Read the model definition and answer for the solid it produces. Units are mm, in the model's axes. Give positions to 0.01 mm unless a question says otherwise; leave off trailing zeros. Order: outer loops, then holes, each group sorted by start corner. A loop starts at its lowest first (then second) coordinate and runs counter-clockwise, first axis right, second up. Notation, with made-up numbers: (85.5, -32) - (127.5, -32) arc R22 cw to (127.5, 2) - close; hole circle Ø9 at (83, 62.25). An arc over 180 degrees is marked (long way). One line per item, written item: value. Start each with the question number.
```python
from build123d import *

# Parameters (mm, degrees)
F1_DEPTH = 76.2


with BuildPart() as f1:
    # F0 (on Top) → F1 (new body)
    with BuildSketch(Plane.XY):
        with BuildLine():
            ThreePointArc((5.0166433221, -50.5516892871), (18.3621332827, -47.3653044043), (30.3681236725, -40.7236671312))
            ThreePointArc((30.3681236725, -40.7236671312), (24.4383893444, -33.8843769742), (21.2835539426, -25.4))
            Line((21.2835539426, -25.4), (-16.2238025261, -25.4))
            ThreePointArc((-16.2238025261, -25.4), (-15.9591486415, -27.5028208782), (-15.8707254658, -29.6203852022))
            ThreePointArc((-15.8707254658, -29.6203852022), (-17.3915692894, -38.277515229), (-21.771977458, -45.8979411038))
            ThreePointArc((-21.771977458, -45.8979411038), (-8.6948058368, -50.050378135), (5.0166433221, -50.5516892871))
        make_face()
    extrude(amount=F1_DEPTH)


solid = f1.part
```
1) Section C-C on y = -37 is taken. Write down the section's boundary in (x, z), plus the area to 3 significant figures.
2) Section B-B on x = 27 is taken. Write down the section's boundary in (y, z).
3) Find the intervals of material crossed by probe 1 along Y at (x, z) = (1, 69); probe 2 along Y at (x, z) = (7, 51.5); probe 3 along X at (y, z) = (-43.75, 28), in increasing order. Write a range as from..to.
4) Section A-A on z = 17 is taken. Write down the section's boundary in (x, y), plus the area to 3 significant figures.
5) Each of these flat-tipped pins is pushed along its axis until it touches: pin 1 (3 mm diameter, centred on y = -32.5, z = 46.5, fed in from -X); pin 2 (1 mm diameter, centred on y = -29.5, z = 68, fed in from +X); pin 3 (3 mm diameter, centred on y = -46.5, z = 25.5, fed in from +X). Where does it stop, or does it pass through?
Solved:
1. outline: (-16.97, 0) - (26.62, 0) - (26.62, 76.2) - (-16.97, 76.2) - close
1. area: 3,320 mm2
2. outline: (-43.03, 0) - (-37.46, 0) - (-37.46, 76.2) - (-43.03, 76.2) - close
3. probe 1: y = -50.79..-25.4
3. probe 2: y = -50.32..-25.4
3. probe 3: x = -20.16..25.82
4. outline: (-21.77, -45.9) arc R50.8 ccw to (30.37, -40.72) arc R25.4 cw to (21.28, -25.4) - (-16.22, -25.4) arc R25.4 cw to start
4. area: 1,010 mm2
5. pin 1: stops at x = -16.25
5. pin 2: stops at x = 22.56
5. pin 3: stops at x = 23.57
